from build123d import *

# Parameters (mm, degrees)
EXTRUDE_1_DEPTH     = 12
SKETCH_2_R          = 1.5
CUT_EXTRUDE_1_DEPTH = 12


with BuildPart() as part:
    # 草图1 → 凸台-拉伸1 (new body)
    with BuildSketch(Plane(origin=(0, 0, 0), x_dir=(1, 0, 0), z_dir=(0, 1, 0))):
        with BuildLine():
            Line((-13, 0), (-8.5, 0))
            ThreePointArc((-8.5, 0), (0, -8.5), (8.5, 0))
            Line((8.5, 0), (13, 0))
            Line((13, 0), (13, -12))
            Line((13, -12), (-13, -12))
            Line((-13, -12), (-13, 0))
        make_face()
    extrude(amount=EXTRUDE_1_DEPTH)

    # 草图2 → 切除-拉伸1 (cut)
    with BuildSketch(Plane.XY.offset(12)):
        with Locations((-11, 3)):
            Circle(SKETCH_2_R)
        with Locations(Location((11, 3, 0), (0, 0, 180))):
            Circle(SKETCH_2_R)
        with Locations((11, 8.999543006)):
            Circle(SKETCH_2_R)
        with Locations(Location((-11, 8.999543006, 0), (0, 0, 180))):
            Circle(SKETCH_2_R)
    extrude(amount=-CUT_EXTRUDE_1_DEPTH, mode=Mode.SUBTRACT)


solid = part.part
Could you check a few things on this model? Use its own coordinates, in mm. Give positions to 0.01 mm unless a question says otherwise; leave off trailing zeros. Order: outer loops, then holes, each group sorted by start corner. A loop starts at its lowest first (then second) coordinate and runs counter-clockwise, first axis right, second up.
1. Suppose I cut it at A-A (y = 3). List the corners of the cut face in (x, z) for me, plus the area to 3 significant figures.
2. Suppose I cut it at D-D (y = 5.75). List the corners of the cut face in (x, z) for me.
3. Will this pin go through, and if not, where does the flat tip stop? P1, Ø1.8, axis at x = 11, y = 9, coming from the -Z side.
4. I need wall thicknesses on L1, parallel to Y at x = 11, z = 9.75; L2, parallel to X at y = 9, z = 11.5; L3, parallel to X at y = 8, z = 9.5. Which ranges of each line are inside material? Lowest first, please.
5. We'd pull the mould along Y, two halves only. Please class faces 1 (the flat face through (0, 12, 9)), 2 (the cylindrical face through (-10.675, 10.464, 6.084)), 3 (the cylindrical face through (-12.2, 2.1, 6.1)), 4 (the flat face through (-11, 6, 0)): pulls with the +Y half, pulls with the -Y half, needs draft (parallel to the pull), parting line crosses it, or undercut.
6. Suppose I cut it at B-B (x = 11). List the corners of the cut face in (y, z) for me.
7. Suppose I cut it at C-C (z = 6.75). List the corners of the cut face in (x, y) for me.
Solved:
1. outline: (-13, 0) - (-12.5, 0) - (-12.5, 12) - (-13, 12) - close; (-9.5, 0) - (-8.5, 0) arc R8.5 cw to (8.5, 0) - (9.5, 0) - (9.5, 12) - (-9.5, 12) - close; (12.5, 0) - (13, 0) - (13, 12) - (12.5, 12) - close
1. area: 127 mm2
2. outline: (-13, 0) - (-8.5, 0) arc R8.5 cw to (8.5, 0) - (13, 0) - (13, 12) - (-13, 12) - close
3. P1: passes through
4. L1: y = 0 to 1.5, 4.5 to 7.5, 10.5 to 12
4. L2: x = -13 to -12.5, -9.5 to 9.5, 12.5 to 13
4. L3: x = -13 to -12.12, -9.88 to 9.88, 12.12 to 13
5. face 1: pulls with the +Y half
5. face 2: undercut
5. face 3: undercut
5. face 4: needs draft
6. outline: (0, 0) - (1.5, 0) - (1.5, 12) - (0, 12) - close; (4.5, 0) - (7.5, 0) - (7.5, 12) - (4.5, 12) - close; (10.5, 0) - (12, 0) - (12, 12) - (10.5, 12) - close
7. outline: (-13, 0) - (-5.17, 0) - (-5.17, 12) - (-13, 12) - close; (5.17, 0) - (13, 0) - (13, 12) - (5.17, 12) - close; hole circle Ø3 at (-11, 3); hole circle Ø3 at (-11, 9); hole circle Ø3 at (11, 3); hole circle Ø3 at (11, 9)
